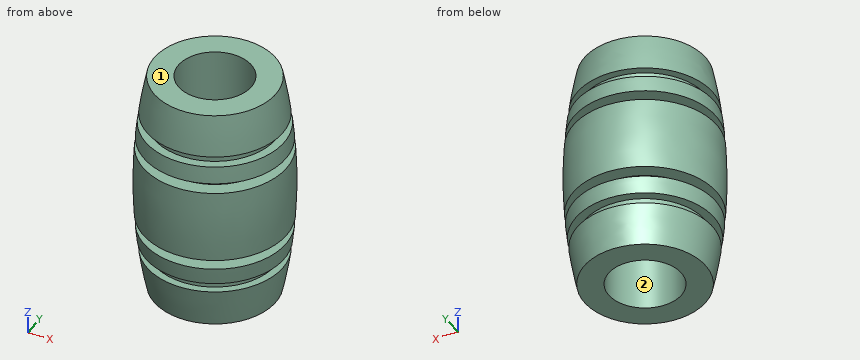
from build123d import *

# Parameters (mm, degrees)
SKETCH4_W   = 1.1
SKETCH4_H   = 1.375
SKETCH4_H_2 = 1.65


with BuildPart() as part:
    # Sketch5 → Revolve1 (revolve)
    with BuildSketch(Plane(origin=(0, 0, 0), x_dir=(0, 0, -1), z_dir=(1, 0, 0))):
        with BuildLine():
            Line((-12.5, 4), (12.5, 4))
            Line((12.5, 4), (12.5, 6.666666667))
            ThreePointArc((12.5, 6.666666667), (0, 8), (-12.5, 6.666666667))
            Line((-12.5, 6.666666667), (-12.5, 4))
        make_face()
    revolve(axis=Axis((0, 0, 12.5), (0, 0, -1)))

    # Sketch4 → Cut-Revolve1 (revolve, cut)
    with BuildSketch(Plane(origin=(0, 0, 0), x_dir=(0, 0, -1), z_dir=(1, 0, 0))):
        with Locations((-7.55, -7.3125)):
            Rectangle(SKETCH4_W, SKETCH4_H)
        with Locations((7.55, -7.3125)):
            Rectangle(SKETCH4_W, SKETCH4_H)
        with Locations((-4.575, -7.175)):
            Rectangle(SKETCH4_W, SKETCH4_H_2)
        with Locations((4.575, -7.175)):
            Rectangle(SKETCH4_W, SKETCH4_H_2)
    revolve(axis=Axis((0, 0, 12.5), (0, 0, -1)), mode=Mode.SUBTRACT)


solid = part.part
CAD build for the part. Positions are in the model's coordinates, mm. Face numbers are marked on the shaded views. Give positions to 0.01 mm unless a question says otherwise; leave off trailing zeros. Answer in a Markdown table with one row per item. Add a question column.
Item 1: Drop flat-ended pins along their axis: P1, Ø4.5, axis at x = -1, y = -0.5, coming from the +Z side; P2, Ø8, axis at x = -2, z = 7.5, coming from the +Y side; P3, Ø1, axis at x = 0.5, z = 1, coming from the +Y side; P4, Ø4, axis at x = 1, z = 2.5, coming from the -Y side. Give the stop position or say it passes through.
Item 2: Probe probe 1 along X at (y, z) = (0, 0.5); probe 2 along Y at (x, z) = (1.75, 2.5); probe 3 along X at (y, z) = (0, 6.25). List the from-to ranges inside material, lowest first.
Item 3: Mould opens along Y. For the marked faces 1 and 2 say: +Y half, -Y half, draft (parallel to the pull), parting line (faces both ways), or undercut.
Reply:
| question | item | result |
|---|---|---|
| 1 | P1 | passes through |
| 1 | P2 | stops at y = 7.87 |
| 1 | P3 | stops at y = 8 |
| 1 | P4 | stops at y = -8 |
| 2 | probe 1 | x = -8 to -4, 4 to 8 |
| 2 | probe 2 | y = -7.75 to -3.6, 3.6 to 7.75 |
| 2 | probe 3 | x = -7.67 to -4, 4 to 7.67 |
| 3 | face 1 | draft |
| 3 | face 2 | undercut |
